Can you work these out from the model? Positions are in its coordinate system, mm. A direction names the side the tool comes from. Give positions to 0.01 mm unless a question says otherwise; leave off trailing zeros. Write each loop counter-clockwise with the first axis right and the second up, starting at its lowest first coordinate (ties: lowest second). Pieces come first, ordered by that corner, then holes. Notation, with made-up numbers: M -19.75,-25.75 L 1.25,-25.75 A21 cw 1.25,13.25 Z; hole C 45.5,18.25 d2. An arc over 180 degrees is marked long. Use CSV: the item, a comma, the result in double quotes. Start each with the question number.
from build123d import *

# Parameters (mm, degrees)
BOSS_EXTRUDE1_DEPTH = 38.1
SKETCH2_R           = 6.35
CUT_EXTRUDE1_DEPTH  = 86.1
SKETCH4_R           = 4.765
CUT_EXTRUDE2_DEPTH  = 9.1


with BuildPart() as part:
    # Sketch1 → Boss-Extrude1 (new body)
    with BuildSketch(Plane.XY):
        with BuildLine():
            Line((0, 0), (44.591, 0))
            ThreePointArc((44.591, 0), (51.329727625, 2.791272375), (54.121, 9.53))
            Line((54.121, 9.53), (54.121, 85.72))
            ThreePointArc((54.121, 85.72), (51.329727625, 92.458727625), (44.591, 95.25))
            Line((44.591, 95.25), (-9.389, 95.25))
            Line((-9.389, 95.25), (-9.389, 101.78))
            Line((-9.389, 101.78), (51.121, 101.78))
            ThreePointArc((51.121, 101.78), (57.859727625, 98.988727625), (60.651, 92.25))
            Line((60.651, 92.25), (60.651, 3))
            ThreePointArc((60.651, 3), (57.859727625, -3.738727625), (51.121, -6.53))
            Line((51.121, -6.53), (-2.37672563, -6.53))
            Line((-2.37672563, -6.53), (-38.738347031, 23.981023107))
            Line((-38.738347031, 23.981023107), (-34.54094394, 28.983293321))
            Line((-34.54094394, 28.983293321), (0, 0))
        make_face()
    extrude(amount=BOSS_EXTRUDE1_DEPTH)

    # Sketch2 → Cut-Extrude1 (cut)
    with BuildSketch(Plane(origin=(0, 101.78, 0), x_dir=(1, 0, 0), z_dir=(0, 1, 0))):
        with Locations(Location((11.421, -19.05, 0), (0, 0, 270))):
            Circle(SKETCH2_R)
    extrude(amount=-CUT_EXTRUDE1_DEPTH, mode=Mode.SUBTRACT)

    # Sketch4 → Cut-Extrude2 (cut)
    with BuildSketch(Plane(origin=(-4.197403091, -5.002270214, 0), x_dir=(0.7660444431189817, -0.642787609686535, 0), z_dir=(-0.642787609686535, -0.7660444431189818, 0))):
        with Locations((-21.356637185, 19.05)):
            Circle(SKETCH4_R)
    extrude(amount=-CUT_EXTRUDE2_DEPTH, mode=Mode.SUBTRACT)


solid = part.part
(1) I want a section at A-A (z = 10). Write out the boundary of the cut face in (x, y), and give its area (3 significant figures).
(2) Please list where these lines run through material, in increasing order: L1, parallel to Y at x = 35, z = 17; L2, parallel to X at y = 68, z = 29; L3, parallel to X at y = 26, z = 13.5. Write a range as [from, to].
(3) Thinking about a two-plate mould opening in Y: for faces 1 (the face through (-24.34, 11.9, 18.78)), 2 (the face through (51.26, 2.72, 18.78)), 3 (the face through (60.651, 48, 19)), 4 (the face through (20, 101.78, 19)), which applies, released by +Y, released by -Y, zero draft, split by the parting line, or undercut?
(4) I want a section at C-C (z = 19.05). Write out the boundary of the cut face in (x, y), and give its area (3 significant figures).
(5) I want a section at B-B (x = 47). Write out the boundary of the cut face in (y, z).
(6) I want a section at D-D (x = 8). Write out the boundary of the cut face in (y, z), and give its area (3 significant figures).
(7) Which directions (+Z, -Z, +X, -X, +Y, -Y) give clear straight access to the entire face, cutting with the end or side of a thin tool? Please do faces 5 (the face through (-9.389, 98, 19)), 6 (the face through (54.121, 47, 19)), 7 (the face through (25, -6.53, 19)), 8 (the face through (18, 95.25, 19)), 9 (the face through (16.78, 98.56, 22.46)).
(8) Will these pins go through, and if not, where does the flat tip stop? pin 1 Ø10 at (x, z) = (11.421, 19.05) entering from +Y; pin 2 Ø3 at (x, z) = (-7.5, 30) entering from -Y; pin 3 Ø7 at (y, z) = (98, 22.5) entering from -X.
Geometry results:
1,outline,"M -38.74,23.98 L -2.38,-6.53 L 51.12,-6.53 A9.53 ccw 60.65,3 L 60.65,92.25 A9.53 ccw 51.12,101.78 L -9.39,101.78 L -9.39,95.25 L 44.59,95.25 A9.53 cw 54.12,85.72 L 54.12,9.53 A9.53 cw 44.59,0 L 0,0 L -34.54,28.98 Z"
1,area,"1,790 mm2"
2,L1,"y = [-6.53, 0], [95.25, 101.78]"
2,L2,"x = [54.12, 60.65]"
2,L3,"x = [-37.04, -30.99], [54.12, 60.65]"
3,face 1,"released by -Y"
3,face 2,"undercut"
3,face 3,"zero draft"
3,face 4,"released by +Y"
4,outline,"M -38.74,23.98 L -24.21,11.79 L -20.01,16.79 L -34.54,28.98 Z; M -16.91,5.66 L -2.38,-6.53 L 51.12,-6.53 A9.53 ccw 60.65,3 L 60.65,92.25 A9.53 ccw 51.12,101.78 L 17.77,101.78 L 17.77,95.25 L 44.59,95.25 A9.53 cw 54.12,85.72 L 54.12,9.53 A9.53 cw 44.59,0 L 0,0 L -12.71,10.66 Z; M -9.39,95.25 L 5.07,95.25 L 5.07,101.78 L -9.39,101.78 Z"
4,area,"1,640 mm2"
5,outline,"M -6.53,0 L 0.31,0 L 0.31,38.1 L -6.53,38.1 Z; M 94.94,0 L 101.78,0 L 101.78,38.1 L 94.94,38.1 Z"
6,outline,"M -6.53,0 L 0,0 L 0,38.1 L -6.53,38.1 Z; M 95.25,0 L 101.78,0 L 101.78,13.7 L 95.25,13.7 Z; M 95.25,24.4 L 101.78,24.4 L 101.78,38.1 L 95.25,38.1 Z"
6,area,"428 mm2"
7,face 5,"+Z, -Z, -X, +Y"
7,face 6,"+Z, -Z"
7,face 7,"+Z, -Z, +X, -X, -Y"
7,face 8,"+Z, -Z, -X"
7,face 9,"+Y"
8,pin 1,"stops at y = 0"
8,pin 2,"stops at y = -3.49"
8,pin 3,"stops at x = -9.39"
